Verification items for the finished model (mm, model axes). Coordinates: 2 decimals unless noted, no trailing zeros. Order: outer loops, then holes, each group sorted by start corner. A loop starts at its lowest first (then second) coordinate and runs counter-clockwise, first axis right, second up. Notation, with made-up numbers: M 15,-3 L 54,-3 A18 ccw 54,17 Z; hole C 23.25,82.25 d1. An arc over 180 degrees is marked long. Answer as a JSON object with one key per item and string values. Group by question number.
(1) Material ranges on line 1 (Y direction, x = 87, z = 1); line 2 (X direction, y = -25.5, z = 1.8); line 3 (Y direction, x = 79.5, z = 0.1), recorded low to high.
(2) Cross-section at C-C (z = 1.5). Enter the section's corners in (x, y).
(3) Cross-section at B-B (y = -24). Enter the section's corners in (x, z), plus the area to 3 significant figures.
(4) Cross-section at A-A (x = 60). Enter the section's corners in (y, z), plus the area to 3 significant figures.
(5) Gauge pin test, flat end, axial feed: pin 1 Ø5.5 at (x, y) = (7, -86.15) entering from +Z. Record the tip position at first contact, or that the pin passes through.
from build123d import *

# Parameters (mm, degrees)
ESQUISSE1_W      = 94
ESQUISSE1_H      = 93
EXTRUSION1_DEPTH = 2
CONG_1_R         = 6.3


with BuildPart() as part:
    # Esquisse1 → Extrusion1 (new body)
    with BuildSketch(Plane.XY):
        with Locations((47, -46.5)):
            Rectangle(ESQUISSE1_W, ESQUISSE1_H)
        with BuildLine():
            Line((88, -10.204101966), (88, -82.795898034))
            ThreePointArc((88, -82.795898034), (89.419273594, -88.67925192), (83.604782776, -87))
            Line((83.604782776, -87), (10.395217224, -87))
            ThreePointArc((10.395217224, -87), (4.580726406, -88.67925192), (6, -82.795898034))
            Line((6, -82.795898034), (6, -10.204101966))
            ThreePointArc((6, -10.204101966), (4.580726406, -4.32074808), (10.395217224, -6))
            Line((10.395217224, -6), (83.604782776, -6))
            ThreePointArc((83.604782776, -6), (89.419273594, -4.32074808), (88, -10.204101966))
        make_face(mode=Mode.SUBTRACT)
    extrude(amount=EXTRUSION1_DEPTH)

    # Congé1
    cong_1_edges = [part.edges().sort_by_distance(p)[0] for p in [
        (0, -93, 1),
        (0, 0, 1),
        (94, 0, 1),
        (94, -93, 1),
    ]]
    fillet(cong_1_edges, radius=CONG_1_R)


solid = part.part
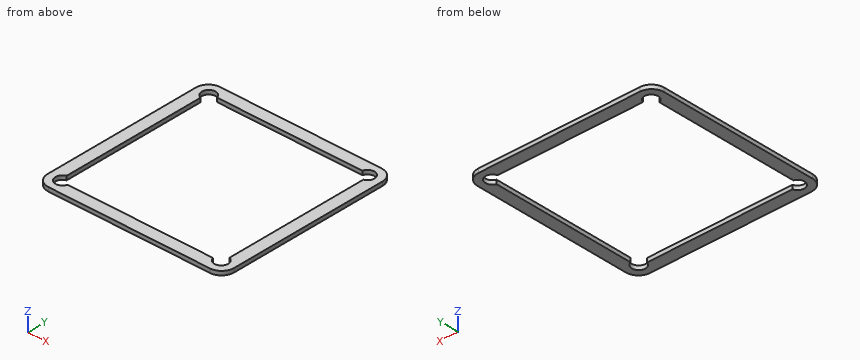
Taken from the geometry:
{
 "1": {"line 1": "y = -93 to -89.65, -3.35 to 0", "line 2": "x = 0 to 6, 88 to 94", "line 3": "y = -93 to -87, -6 to 0"},
 "2": {"outline": "M 0,-86.7 A6.3 ccw 6.3,-93 L 87.7,-93 A6.3 ccw 94,-86.7 L 94,-6.3 A6.3 ccw 87.7,0 L 6.3,0 A6.3 ccw 0,-6.3 Z; hole M 6,-82.8 A3.5 ccw long 10.4,-87 L 83.6,-87 A3.5 ccw long 88,-82.8 L 88,-10.2 A3.5 ccw long 83.6,-6 L 10.4,-6 A3.5 ccw long 6,-10.2 Z"},
 "3": {"outline": "M 0,0 L 6,0 L 6,2 L 0,2 Z; M 88,0 L 94,0 L 94,2 L 88,2 Z", "area": "24.0 mm²"},
 "4": {"outline": "M -93,0 L -87,0 L -87,2 L -93,2 Z; M -6,0 L 0,0 L 0,2 L -6,2 Z", "area": "24.0 mm²"},
 "5": {"pin 1": "passes through"}
}
